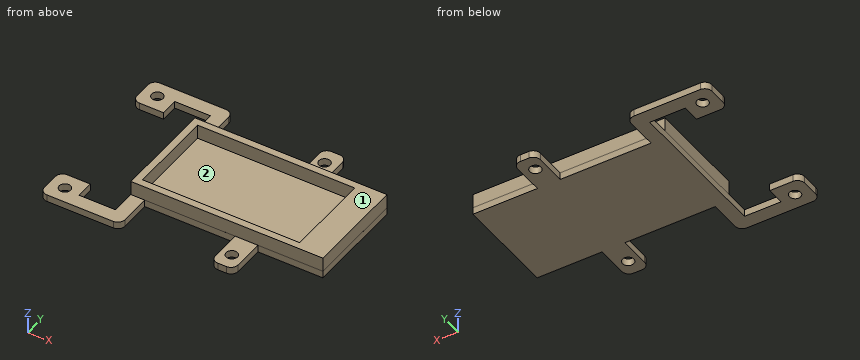
```python
from build123d import *

# Parameters (mm, degrees)
SKETCH_R      = 1.6
PAD_DEPTH     = 2
SKETCH001_W   = 53.9946
SKETCH001_H   = 28.4007
SKETCH001_W_2 = 44.2
SKETCH001_H_2 = 24.4007
PAD001_DEPTH  = 4
FILLET_R      = 2


with BuildPart() as part:
    # Sketch → Pad (new body)
    with BuildSketch(Plane.XY):
        Polygon((21.7667, -25.4923), (21.7667, -16.53082), (30.29072, -16.53082), (30.29072, -21.52783), (40.54589, -21.52783), (40.54589, 20.48012), (30.54589, 20.48012), (30.54589, 15.49558), (21.7928, 15.49558), (21.7928, 24.4708), (44.46409, 24.4708), (44.46409, 13.68925), (70.02404, 13.68925), (70.02404, 24.4708), (76.4105, 24.4708), (76.4105, 13.68925), (94.54589, 13.68925), (94.54589, -14.71075), (76.26045, -14.71075), (76.26045, -25.4923), (69.87399, -25.4923), (69.87399, -14.71075), (44.43799, -14.71075), (44.43799, -25.4923), align=None)
        with Locations((25.98991, 19.9708)):
            Circle(SKETCH_R, mode=Mode.SUBTRACT)
        with Locations((25.99838, -21.01867)):
            Circle(SKETCH_R, mode=Mode.SUBTRACT)
        with Locations((72.97054, 20.01877)):
            Circle(SKETCH_R, mode=Mode.SUBTRACT)
        with Locations((72.94754, -21.05239)):
            Circle(SKETCH_R, mode=Mode.SUBTRACT)
    extrude(amount=PAD_DEPTH)

    # Sketch001 → Pad001 (new body)
    with BuildSketch(Plane.XY.offset(2)):
        with Locations((67.5478, -0.51015)):
            Rectangle(SKETCH001_W, SKETCH001_H)
        with Locations((64.6505, -0.51015)):
            Rectangle(SKETCH001_W_2, SKETCH001_H_2, mode=Mode.SUBTRACT)
    extrude(amount=PAD001_DEPTH)

    # Fillet
    fillet_edges = [part.edges().sort_by_distance(p)[0] for p in [
        (21.7667, -16.53082, 1),
        (21.7667, -25.4923, 1),
        (44.43799, -25.4923, 1),
        (69.87399, -25.4923, 1),
        (76.26045, -25.4923, 1),
        (76.4105, 24.4708, 1),
        (70.02404, 24.4708, 1),
        (44.46409, 24.4708, 1),
        (21.7928, 24.4708, 1),
        (21.7928, 15.49558, 1),
    ]]
    fillet(fillet_edges, radius=FILLET_R)


solid = part.part
```
The model under review builds one solid part; all positions refer to its coordinate system, in mm. Face numbers are marked on the shaded views. Give positions to 0.01 mm unless a question says otherwise; leave off trailing zeros. Write each loop counter-clockwise with the first axis right and the second up, starting at its lowest first coordinate (ties: lowest second). Pieces come first, ordered by that corner, then holes. Notation, with made-up numbers: M -18,53.25 L 4,53.25 A23 ccw 4,78.25 Z; hole C 58,-35.75 d6. An arc over 180 degrees is marked long. Write each question's results on one line, items separated by ' | '. Start each with the question number.
1. Insertion check: pin 1 Ø7.5 at (x, y) = (61, -0.5) entering from +Z; pin 2 Ø1.6 at (y, z) = (-20, 1) entering from +X; pin 3 Ø2 at (x, z) = (63.5, 4) entering from -Y; pin 4 Ø5 at (x, y) = (37, 10) entering from -Z. Each pin has a flat end and moves straight along its axis. Give the tip position at first contact, or say it passes through.
2. We need section B-B (z = 4.35). Write out the cut boundary in (x, y).
3. For probe 1 along X at (y, z) = (22.5, 1.8); probe 2 along Y at (x, z) = (79.5, 5.45); probe 3 along X at (y, z) = (0, 4.75), list the stretches that pass through material, from the lowest coordinate up. Write a range as [from, to].
4. We need section A-A (x = 34). Write out the cut boundary in (y, z).
5. Mouldability with a two-part tool opening along Y and no side actions: class the marked faces 1 and 2 as released by +Y, released by -Y, zero draft, split by the parting line, or undercut.
Results found:
1) pin 1: stops at z = 2 | pin 2: stops at x = 76.26 | pin 3: stops at y = -14.71 | pin 4: passes through
2) outline: M 40.55,-14.71 L 94.55,-14.71 L 94.55,13.69 L 40.55,13.69 Z; hole M 42.55,-12.71 L 86.75,-12.71 L 86.75,11.69 L 42.55,11.69 Z
3) probe 1: x = [21.79, 44.46], [70.02, 76.41] | probe 2: y = [-14.71, -12.71], [11.69, 13.69] | probe 3: x = [40.55, 42.55], [86.75, 94.55]
4) outline: M -25.49,0 L -21.53,0 L -21.53,2 L -25.49,2 Z; M 20.48,0 L 24.47,0 L 24.47,2 L 20.48,2 Z
5) face 1: zero draft | face 2: undercut
